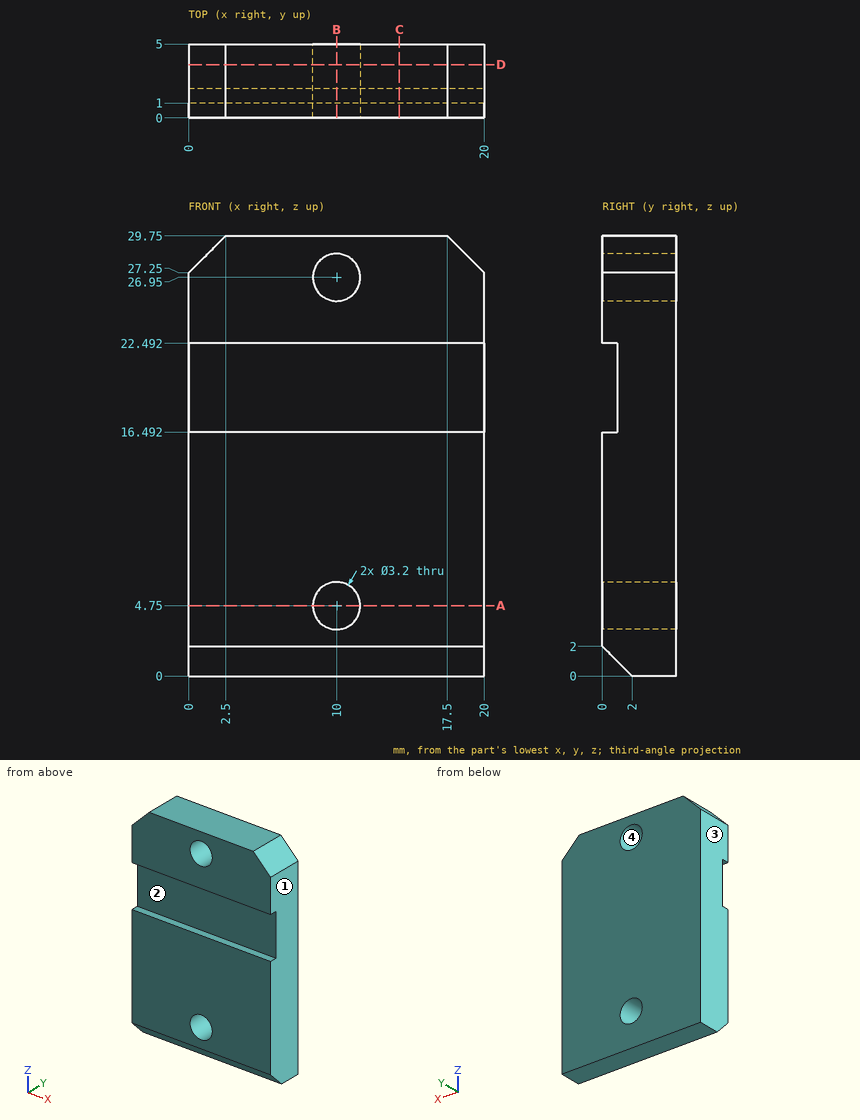
Part print with two shaded views. Sizes in mm from the minimum x, y, z corner. Coordinates: 2 decimals unless noted, no trailing zeros. Order: outer loops, then holes, each group sorted by start corner. A loop starts at its lowest first (then second) coordinate and runs counter-clockwise, first axis right, second up.
(1) Saw through at D-D, the plane y = 3.6. Write the cut outline in (x, z), and give its area (3 significant figures).
Solution:
outline: (0, 0) - (20, 0) - (20, 27.25) - (17.5, 29.75) - (2.5, 29.75) - (0, 27.25) - close; hole circle Ø3.2 at (10, 4.75); hole circle Ø3.2 at (10, 26.95)
area: 573 mm2
(2) Saw through at B-B, the plane x = 10. Write the cut outline in (y, z).
Solution:
outline: (0, 2) - (2, 0) - (5, 0) - (5, 3.15) - (0, 3.15) - close; (0, 6.35) - (5, 6.35) - (5, 25.35) - (0, 25.35) - (0, 22.49) - (1, 22.49) - (1, 16.49) - (0, 16.49) - close; (0, 28.55) - (5, 28.55) - (5, 29.75) - (0, 29.75) - close
(3) Pin check, flat tips, straight feed: pin 1 Ø2 at (x, z) = (7.5, 18.5) entering from -Y; pin 2 Ø1.1 at (x, y) = (9.5, 0.5) entering from -Z. Stop position of each tip, or through.
Solution:
pin 1: stops at y = 1
pin 2: stops at z = 0.95
(4) Mould opens along X. For the marked faces 1, 2, 3 and 4 say: released by +X, released by -X, zero draft, split by the parting line, or undercut.
Solution:
face 1: released by +X
face 2: zero draft
face 3: released by -X
face 4: undercut
(5) Drill centre lines: L1, parallel to Z at x = 10, y = 3.2; L2, parallel to Z at x = 10, y = 1.8; L3, parallel to X at y = 3.55, z = 26.95. Where is each one in solid material? Low to high.
Solution:
L1: z = 0 to 3.15, 6.35 to 25.35, 28.55 to 29.75
L2: z = 0.2 to 3.15, 6.35 to 25.35, 28.55 to 29.75
L3: x = 0 to 8.4, 11.6 to 20
(6) Saw through at A-A, the plane z = 4.75. Write the cut outline in (x, y).
Solution:
outline: (0, 0) - (8.4, 0) - (8.4, 5) - (0, 5) - close; (11.6, 0) - (20, 0) - (20, 5) - (11.6, 5) - close
(7) Saw through at C-C, the plane x = 14.25. Write the cut outline in (y, z), and give its area (3 significant figures).
Solution:
outline: (0, 2) - (2, 0) - (5, 0) - (5, 29.75) - (0, 29.75) - (0, 22.49) - (1, 22.49) - (1, 16.49) - (0, 16.49) - close
area: 141 mm2
